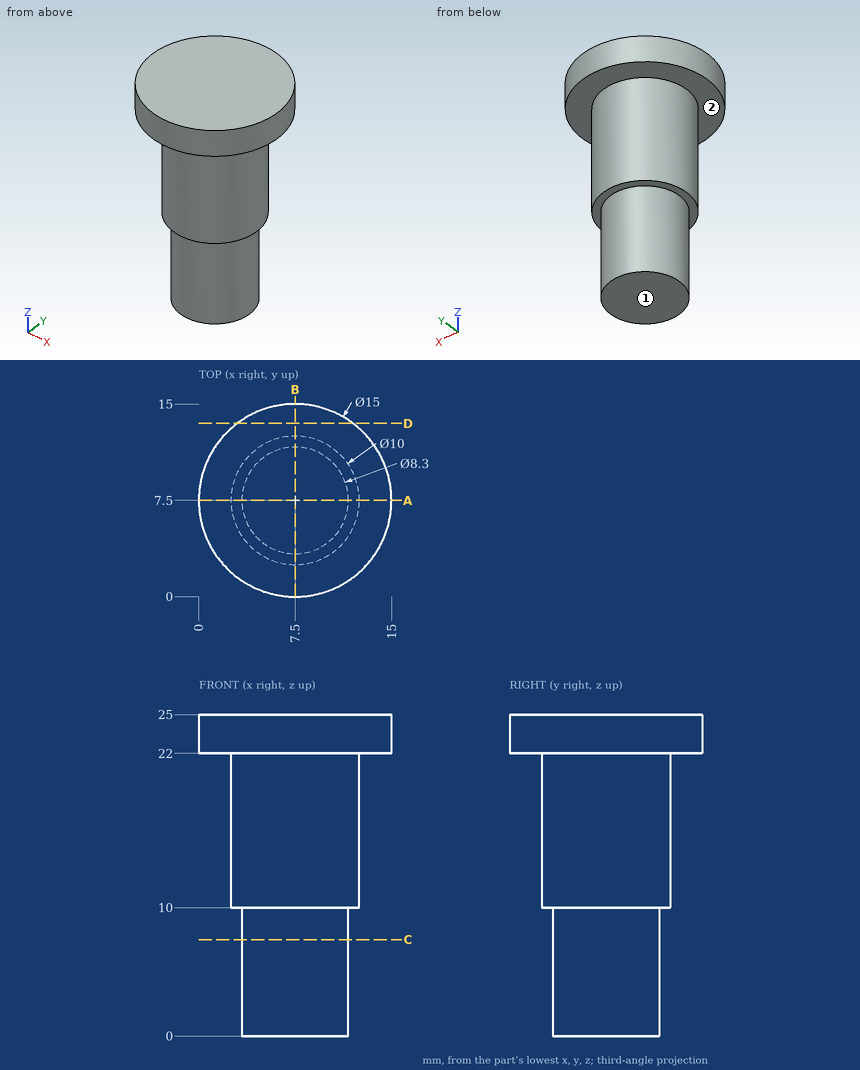
The drawing under review shows one solid part. Ordinate dimensions are in mm from its lowest x, y, z. A direction names the side the tool comes from. Coordinates: 2 decimals unless noted, no trailing zeros. Write each loop counter-clockwise with the first axis right and the second up, starting at its lowest first coordinate (ties: lowest second). Pieces come first, ordered by that corner, then holes. Notation, with made-up numbers: (84.5, -28) - (94.5, -28) arc R19 cw to (94.5, -15) - close; hole circle Ø3 at (65, -9.75). An arc over 180 degrees is marked (long way). Put each result on its own line as item: value.
1. Add section D-D, the plane y = 13.5. Give the boundary of the cut face in (x, z).
Values found:
outline: (3, 22) - (12, 22) - (12, 25) - (3, 25) - close
2. Add section C-C, the plane z = 7.5. Give the boundary of the cut face in (x, y), then the cut area to 3 significant figures.
Values found:
outline: circle Ø8.3 at (7.5, 7.5)
area: 54.1 mm²
3. Wall thickness on probe 1 along Z at (x, y) = (2.5, 11); probe 2 along X at (y, z) = (10.75, 21.25); probe 3 along Y at (x, z) = (11.25, 5.5): over which ranges is each line inside the solid? List them lowest first.
Values found:
probe 1: 22 to 25
probe 2: 3.7 to 11.3
probe 3: 5.72 to 9.28
4. For pin 1 (1.5 mm diameter, centred on y = 12.5, z = 15.5, fed in from -X); pin 2 (3 mm diameter, centred on y = 4, z = 5.5, fed in from -X); pin 3 (3 mm diameter, centred on y = 4.5, z = 20, fed in from -X), all flat-tipped, find the tip position at first contact; note any pin that passes through.
Values found:
pin 1: x = 4.87
pin 2: x = 3.86
pin 3: x = 2.73
5. Add section A-A, the plane y = 7.5. Give the boundary of the cut face in (x, z).
Values found:
outline: (0, 22) - (2.5, 22) - (2.5, 10) - (3.35, 10) - (3.35, 0) - (11.65, 0) - (11.65, 10) - (12.5, 10) - (12.5, 22) - (15, 22) - (15, 25) - (0, 25) - close
6. Machinability: for the marked faces 1 and 2, which of the approach directions +Z, -Z, +X, -X, +Y, -Y give a long, thin tool a straight path to every point of the face, cutting with its end or side? Answer none if there is none.
Values found:
face 1: -Z, +X, -X, +Y, -Y
face 2: -Z
